```python
from build123d import *

# Parameters (mm, degrees)
F3_T2_ANGLE = 212.1305431318
F3_T4_ANGLE = 212.1305431318
F3_T6_ANGLE = 237.3879219603
F3_T8_ANGLE = 237.3879219603


# Not quite as in the source:
# - a fillet or chamfer that OpenCascade refuses, or shapes differently, is made with other operations: its cross-section is extruded or revolved along the edge and cut away or added


with BuildPart() as f2:
    # F2: sweep along a path in F0
    with BuildLine(Plane.XZ) as f2_path:
        ThreePointArc((-12.7, 0), (0, 12.7), (12.7, 0))
    # F1 (on Top) → F2 (sweep)
    with BuildSketch(Plane.XY):
        with BuildLine():
            Line((-12.7, -4.572), (-12.7, 0))
            Line((-12.7, 0), (-22.225, 0))
            Line((-22.225, 0), (-22.225, -2.032))
            Line((-22.225, -2.032), (-20.701, -2.032))
            Line((-20.701, -2.032), (-20.701, -1.651))
            Line((-20.701, -1.651), (-14.732, -1.651))
            Line((-14.732, -1.651), (-14.732, -2.921))
            Line((-14.732, -2.921), (-20.5930953096, -2.921))
            ThreePointArc((-20.5930953096, -2.921), (-20.6693954479, -2.8893954479), (-20.701, -2.8130953096))
            Line((-20.701, -2.8130953096), (-20.701, -2.54))
            Line((-20.701, -2.54), (-22.225, -2.54))
            Line((-22.225, -2.54), (-22.225, -4.572))
            Line((-22.225, -4.572), (-12.7, -4.572))
        make_face()
    sweep(path=f2_path.line)

    # F3: fillet of radius 2.54 on 4 edges, made by hand

    # F3_s1 → F3_t2 (revolve, cut)
    with BuildSketch(Plane(origin=(0, 0, 0), x_dir=(0, 1, 0), z_dir=(0.2767322496, 0, -0.9609470651))):
        with BuildLine():
            ThreePointArc((-2.54, -22.225), (-3.9994755399, -21.3427554727), (-4.572, -19.7363184213))
            Line((-4.572, -19.7363184213), (-4.572, -22.225))
            Line((-4.572, -22.225), (-2.54, -22.225))
        make_face()
    revolve(axis=Axis((0, -4.572, 0), (0, 1, 0)), revolution_arc=F3_T2_ANGLE, mode=Mode.SUBTRACT)

    # F3_s3 → F3_t4 (revolve, cut)
    with BuildSketch(Plane(origin=(0, 0, 0), x_dir=(0, 1, 0), z_dir=(0.2767322496, 0, -0.9609470651))):
        with BuildLine():
            ThreePointArc((0, -19.7363184213), (-0.5725244601, -21.3427554727), (-2.032, -22.225))
            Line((-2.032, -22.225), (0, -22.225))
            Line((0, -22.225), (0, -19.7363184213))
        make_face()
    revolve(axis=Axis((0, 0, 0), (0, 1, 0)), revolution_arc=F3_T4_ANGLE, mode=Mode.SUBTRACT)

    # F3_s5 → F3_t6 (revolve, cut)
    with BuildSketch(Plane(origin=(0, 0, 0), x_dir=(0, 1, 0), z_dir=(0.4801310429, 0, -0.8771967748))):
        with BuildLine():
            ThreePointArc((-2.032, -12.7), (-3.8280512242, -13.4439487758), (-4.572, -15.24))
            Line((-4.572, -15.24), (-4.572, -12.7))
            Line((-4.572, -12.7), (-2.032, -12.7))
        make_face()
    revolve(axis=Axis((0, -4.572, 0), (0, 1, 0)), revolution_arc=F3_T6_ANGLE, mode=Mode.SUBTRACT)

    # F3_s7 → F3_t8 (revolve, cut)
    with BuildSketch(Plane(origin=(0, 0, 0), x_dir=(0, 1, 0), z_dir=(0.4801310429, 0, -0.8771967748))):
        with BuildLine():
            ThreePointArc((-2.54, -12.7), (-0.7439487758, -13.4439487758), (0, -15.24))
            Line((0, -15.24), (0, -12.7))
            Line((0, -12.7), (-2.54, -12.7))
        make_face()
    revolve(axis=Axis((0, 0, 0), (0, 1, 0)), revolution_arc=F3_T8_ANGLE, mode=Mode.SUBTRACT)


solid = f2.part
```
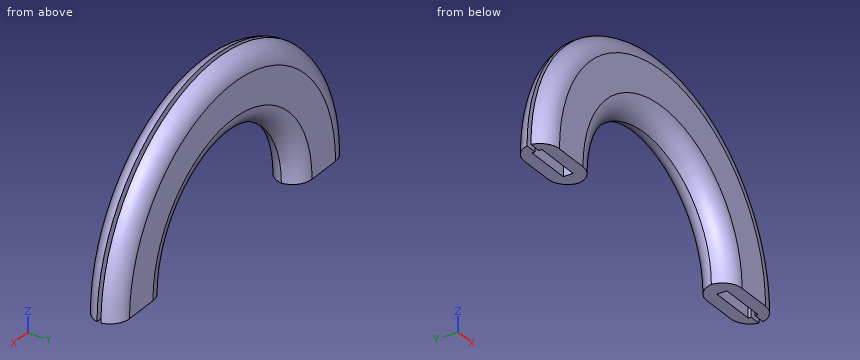
Input: part model. Units: mm. Frame: model coordinates. Round coordinates to 2 decimals unless told otherwise and drop trailing zeros. Loops run counter-clockwise (first coordinate to the right, second up) from the corner with the lowest first, then second, coordinate; pieces in that order, holes last.
1) Section query C-C on y = -0.7. Return the cut outline in (x, z).
Ans:
outline: (-21.49, 0) - (-13.49, 0) arc R13.49 cw to (13.49, 0) - (21.49, 0) arc R21.49 ccw to start
2) Material intervals for line 1 (Y direction, x = 14, z = 13.25); line 2 (Y direction, x = 1, z = 21.25); line 3 (Z direction, x = -2, y = -2.8), sorted ascending.
Ans:
line 1: y = -4.57 to -2.92, -1.65 to 0
line 2: y = -4.05 to -2.54, -2.03 to -0.52
line 3: z = 12.66 to 14.6, 20.6 to 22.07
3) Section query A-A on x = 0. Return the cut outline in (y, z) (3 decimals), plus the area to 3 significant figures.
Ans:
outline: (-4.572, 15.24) arc R2.54 ccw to (-2.286, 12.713) arc R2.54 ccw to (0, 15.24) - (0, 19.736) arc R2.54 ccw to (-2.032, 22.225) - (-2.032, 20.701) - (-1.651, 20.701) - (-1.651, 14.732) - (-2.921, 14.732) - (-2.921, 20.593) arc R0.108 cw to (-2.813, 20.701) - (-2.54, 20.701) - (-2.54, 22.225) arc R2.54 ccw to (-4.572, 19.736) - close
area: 29.9 mm2
4) Pin query (flat end, axial travel): pin 1 (10 mm diameter, centred on x = 0.5, z = 15, fed in from -Y); pin 2 (3 mm diameter, centred on x = -1, z = 11, fed in from -Y); pin 3 (1.5 mm diameter, centred on x = -2, y = -2, fed in from -Z); pin 4 (1.5 mm diameter, centred on y = -1.5, z = 5.5, fed in from +X). Return the tip coordinate at first contact, or that it passes through.
Ans:
pin 1: stops at y = -4.57
pin 2: passes through
pin 3: stops at z = 12.42
pin 4: stops at x = 21.66
5) Section query B-B on y = -3.7. Return the cut outline in (x, z).
Ans:
outline: (-21.65, 0) - (-13.32, 0) arc R13.32 cw to (13.32, 0) - (21.65, 0) arc R21.65 ccw to start
